Solid Edge part; units mm, degrees
sketch "Sketch1" plane through (0, 0, 0) normal (1, 0, 0) x (0, 1, 0)
  line L0 (0, -2.54) -> (0, 2.54)
  arc A0 (0, 2.54) -> (8.255, -2.54) centre (-0.5525, -7.605) cw
  line L1 (0, -2.54) -> (8.255, -2.54)
revolve "RevolvedProtrusion1" add sketch "Sketch1" angle 360 about axis through (0, 0, -14.7796) along (0, 0, 1)
sketch "Sketch2" plane through (0, 0, -2.54) normal (0, 0, -1) x (0, 1, 0)
  circle A0 centre (0, 0) radius 4.7625
extrude "Protrusion1" add sketch "Sketch2" along normal blind 19.05
sketch "Sketch3" plane through (0, 0, -21.59) normal (0, 0, -1) x (1, 0, 0)
  circle A0 centre (0, 0) radius 4.76
extrude "Cutout1" cut sketch "Sketch3" against normal blind 17.4625 flip side to cut
sketch "Sketch4" plane through (-0.6032, 0.3606, 5.08) normal (0, 0, 1) x (1, 0, 0)
  line L0 (-1.0007, 2.4175) -> (2.2072, 2.4175)
  line L1 (3.8111, -0.3606) -> (2.2072, 2.4175)
  line L2 (2.2072, -3.1387) -> (3.8111, -0.3606)
  line L3 (-1.0007, -3.1387) -> (2.2072, -3.1387)
  line L4 (-2.6047, -0.3606) -> (-1.0007, -3.1387)
  line L5 (-1.0007, 2.4175) -> (-2.6047, -0.3606)
extrude "ExtrudedCutout_11" cut sketch "Sketch4" against normal blind 7.62
properties part number "163737"
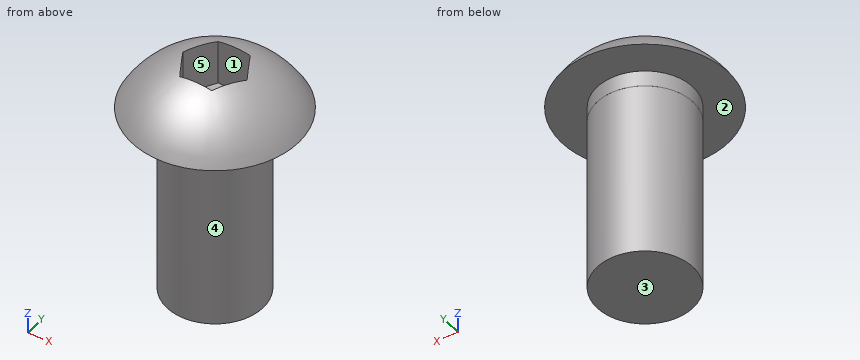
Build history of the part. All positions in model axes, mm. Face numbers are marked on the shaded views. A direction names the side the tool comes from. Round coordinates to 2 decimals unless told otherwise and drop trailing zeros. Write each loop counter-clockwise with the first axis right and the second up, starting at its lowest first coordinate (ties: lowest second). Pieces come first, ordered by that corner, then holes. Notation, with made-up numbers: (-5.75, 50.25) -> (7.25, 50.25) arc R20 ccw to (7.25, 73.25) -> close; hole circle Ø7 at (48, -34.75). An arc over 180 degrees is marked (long way). Write item = value, one per line.
(1) Probe L1, parallel to Z at x = 2, y = -1.5; L2, parallel to X at y = -0.25, z = -12.75; L3, parallel to X at y = -4.25, z = -8.25. List the from-to ranges inside material, lowest first.
Answer:
L1 = -21.59 to -2.54
L2 = -4.75 to 4.75
L3 = -2.14 to 2.14
(2) Flat gauge pins, fed straight in: pin 1 (2 mm diameter, centred on x = 4, y = 3.5, fed in from -Z); pin 2 (1 mm diameter, centred on x = 0.5, y = 5.5, fed in from -Z); pin 3 (1.5 mm diameter, centred on x = 0, z = -18.5, fed in from +Y); pin 4 (8 mm diameter, centred on x = -5, z = -8, fed in from -Y). Where does each tip first touch, or does it go through?
Answer:
pin_1 = -21.59
pin_2 = -2.54
pin_3 = 4.76
pin_4 = -4.65
(3) Band-saw the part on A-A (z = -14.75). Give the cut face in (x, y), then the cut area to 3 significant figures.
Answer:
outline = circle Ø9.52 at (0, 0)
area = 71.2 mm2
(4) Tool access for the marked faces 1 and 2: list every direction of +Z, -Z, +X, -X, +Y, -Y with a clear straight run to the whole face (end or side of a thin tool).
Answer:
face_1 = +Z
face_2 = -Z
(5) Two-plate mould, pull along X, no slides. Class the marked faces 3, 4 and 5: pulls with the +X half, pulls with the -X half, needs draft (parallel to the pull), parting line crosses it, or undercut.
Answer:
face_3 = needs draft
face_4 = parting line crosses it
face_5 = undercut
